Autodesk Inventor part; units mm, degrees
ref_plane "YZ Plane" through (0, 0, 0) normal (1, 0, 0) x (0, 1, 0)
ref_plane "XZ Plane" through (0, 0, 0) normal (0, 1, 0) x (-1, 0, 0)
ref_plane "XY Plane" through (0, 0, 0) normal (0, 0, 1) x (1, 0, 0)
sketch "Sketch1" plane through (0, 0, 0) normal (0, 0, 1) x (1, 0, 0)
  line L0 (-177.8, -31.75) -> (177.8, -31.75)
  line L1 (177.8, -31.75) -> (177.8, 31.75)
  line L2 (177.8, 31.75) -> (-177.8, 31.75)
  line L3 (-177.8, 31.75) -> (-177.8, -31.75)
  line L4 (-177.8, -31.75) -> (177.8, 31.75) construction
  line L5 (177.8, -31.75) -> (-177.8, 31.75) construction
  point P0 (0, 0)
  point P1 (0, 0)
  dimension "d31" = 355.6
  dimension "d32" = 63.5
extrude "Plate1" add sketch "Sketch1" along normal blind 6.35
sketch "Sketch3" plane through (177.8, -37.3716, 8.6786) normal (0, -0.7071068, -0.7071068) x (1, 0, 0)
  line L0 (-355.6, 0) -> (0, 0)
  line L1 (0, 0) -> (0, 150.7998)
  line L2 (0, 150.7998) -> (-355.6, 150.7998)
  line L3 (-355.6, 150.7998) -> (-355.6, 0)
edge flange "Flange2" height 165.1 angle 45 thickness 6.35 bend radius 7.9502 thickness toward (0, -0.7071068, -0.7071068) relief tear relief width 6.35 relief depth 3.175 edges at (0, -31.75, 6.35) wall of the first edge with corners at (-177.8, -37.3716, 8.6786) (177.8, -37.3716, 8.6786) (177.8, -144.0032, 115.3101) (-177.8, -144.0032, 115.3101)
bend "Bend2"
corner "Corner2"
fillet "Corner Round1" radius 6.35 2 edges at (177.8, 31.75, 3.175) (-177.8, 31.75, 3.175)
fillet "Corner Round2" radius 38.1 2 edges at (177.8, -146.2483, 113.0651) (-177.8, -146.2483, 113.0651)
sketch "Sketch4" plane through (-177.8, -37.3716, 8.6786) normal (0, 0.7071068, 0.7071068) x (1, 0, 0)
  line L0 (152.4, -17.4498) -> (203.2, -17.4498)
  line L1 (215.9, -30.1498) -> (215.9, -115.8748)
  line L2 (203.2, -128.5748) -> (152.4, -128.5748)
  line L3 (139.7, -115.8748) -> (139.7, -30.1498)
  line L4 (139.7, -17.4498) -> (215.9, -128.5748) construction
  line L5 (215.9, -17.4498) -> (139.7, -128.5748) construction
  line L6 (38.1, -150.7998) -> (317.5, -150.7998) construction
  arc A0 (152.4, -17.4498) -> (139.7, -30.1498) centre (152.4, -30.1498) ccw
  arc A1 (215.9, -30.1498) -> (203.2, -17.4498) centre (203.2, -30.1498) ccw
  arc A2 (203.2, -128.5748) -> (215.9, -115.8748) centre (203.2, -115.8748) ccw
  arc A3 (139.7, -115.8748) -> (152.4, -128.5748) centre (152.4, -115.8748) ccw
  line L7 (63.5, -98.4123) -> (63.5, -47.6123) construction
  line L8 (50.8, -98.4123) -> (50.8, -47.6123)
  line L9 (76.2, -47.6123) -> (76.2, -98.4123)
  arc A4 (50.8, -98.4123) -> (76.2, -98.4123) centre (63.5, -98.4123) ccw
  arc A5 (76.2, -47.6123) -> (50.8, -47.6123) centre (63.5, -47.6123) ccw
  line L10 (0, -112.6998) -> (0, 0)
  line L11 (177.8, -73.0123) -> (177.8, -150.7998) construction
  line L12 (292.1, -98.4123) -> (292.1, -47.6123) construction
  line L13 (304.8, -98.4123) -> (304.8, -47.6123)
  line L14 (279.4, -47.6123) -> (279.4, -98.4123)
  arc A6 (279.4, -98.4123) -> (304.8, -98.4123) centre (292.1, -98.4123) ccw
  arc A7 (304.8, -47.6123) -> (279.4, -47.6123) centre (292.1, -47.6123) ccw
  point P0 (63.5, -73.0123)
  dimension "d45" = 22.225
  dimension "d46" = 76.2
  dimension "d47" = 111.125
  dimension "d50" = 12.7
  dimension "d51" = 12.7
  dimension "d52" = 50.8
  dimension "d53" = 63.5
  dimension "d54" = 25.4
extrude "Cut1" cut sketch "Sketch4" against normal blind 6.35
equation "\"d48\" = Thickness"
equation "\"d15\" = Thickness"
equation "\"d33\" = BendReliefWidth"
equation "\"d34\" = BendReliefDepth"
equation "\"d35\" = MinimumRemnant"
equation "\"d36\" = TransitionRadius"
equation "\"d39\" = BendRadius"
equation "\"d40\" = CornerReliefSize"
equation "\"d41\" = GapSize"
equation "\"d42\" = JacobiRadiusSize"
equation "\"BendReliefWidth\" = Thickness"
equation "\"BendReliefDepth\" = 0.5 * Thickness"
equation "\"CornerReliefSize\" = 4 * Thickness"
equation "\"MinimumRemnant\" = 2 * Thickness"
equation "\"TransitionRadius\" = BendRadius"
equation "\"JacobiRadiusSize\" = Thickness"
equation "\"GapSize\" = Thickness"
properties part number "Model-4_Sheet Stifferner" material "SS304"
Verification items for the finished model (mm, model axes). A direction names the side the tool comes from. Give positions to 0.01 mm unless a question says otherwise; leave off trailing zeros. Write each loop counter-clockwise with the first axis right and the second up, starting at its lowest first coordinate (ties: lowest second). Pieces come first, ordered by that corner, then holes. Notation, with made-up numbers: M -39.75,89.25 L 12.25,89.25 A25 cw 12.25,105.25 Z; hole C -7,78 d9. An arc over 180 degrees is marked long. Write item = value, one per line.
(1) Sectioned sample at D-D (y = 19). Record the cut outline in (x, z).
Found:
outline = M -177.8,0 L 177.8,0 L 177.8,6.35 L -177.8,6.35 Z
(2) Material ranges on line 1 (X direction, y = -65, z = 32.5); line 2 (Z direction, x = -45.5, y = -14); line 3 (Y direction, x = -158.5, z = 14), recorded low to high.
Found:
line_1 = -177.8 to -120.23, -108.37 to -38.1, 38.1 to 108.37, 120.23 to 177.8
line_2 = 0 to 6.35
line_3 = -51.67 to -42.69
(3) Sectioned sample at A-A (x = -21). Record the cut outline in (y, z).
Found:
outline = M -148.49,110.82 L -132.78,95.1 L -128.29,99.59 L -144,115.31 Z; M -54.2,16.53 L -41.86,4.19 A14.3 ccw -31.75,0 L 31.75,0 L 31.75,6.35 L -31.75,6.35 A7.95 cw -37.37,8.68 L -49.71,21.02 Z
(4) Sectioned sample at B-B (x = 134). Record the cut outline in (y, z), then the cut area to 3 significant figures.
Found:
outline = M -148.49,110.82 L -41.86,4.19 A14.3 ccw -31.75,0 L 31.75,0 L 31.75,6.35 L -31.75,6.35 A7.95 cw -37.37,8.68 L -144,115.31 Z
area = 1,420 mm2
(5) Draft check along X on faces 4 (the face through (101.6, -91, 58)), 5 (the face through (-177.8, -54, 25)), 6 (the face through (-2, 0, 6.35)). Enter one of: released by +X, released by -X, zero draft, split by the parting line, or undercut.
Found:
face_4 = undercut
face_5 = released by -X
face_6 = zero draft
(6) Go/stop test with flat-tipped pins: pin 1 Ø1 at (x, z) = (-95.5, 56) entering from -Y; pin 2 Ø6 at (x, z) = (-64, 39) entering from -Y; pin 3 Ø2 at (x, y) = (-42, -44.5) entering from +Z; pin 4 Ø20 at (y, z) = (-97, 54) entering from -X. Record where each tip stops, or that it passes through.
Found:
pin_1 = -94.17
pin_2 = -79.67
pin_3 = 16.81
pin_4 = -177.8
(7) Sectioned sample at C-C (z = 52.5). Record the cut outline in (x, y), then the cut area to 3 significant figures.
Found:
outline = M -177.8,-90.17 L -127,-90.17 L -127,-81.19 L -177.8,-81.19 Z; M -101.6,-90.17 L -38.1,-90.17 L -38.1,-81.19 L -101.6,-81.19 Z; M 38.1,-90.17 L 101.6,-90.17 L 101.6,-81.19 L 38.1,-81.19 Z; M 127,-90.17 L 177.8,-90.17 L 177.8,-81.19 L 127,-81.19 Z
area = 2,050 mm2
(8) Access from +Z, -Z, +X, -X, +Y, -Y to the whole of each face (thin tool, end or side, straight path). Record for faces 1 (the face through (-34.281, -54.485, 21.365)), 2 (the face through (34.28, -127.94, 94.82)), 3 (the face through (-175.89, 29.94, 3.22)).
Found:
face_1 = +Z, -Y
face_2 = -Z, +Y
face_3 = +Z, -Z, -X, +Y
